```python
from build123d import *

# Parameters (mm, degrees)
SKETCH_W         = 90
SKETCH_H         = 64
PAD_DEPTH        = 2
HOLE_D           = 2.9
HOLE_DEPTH       = 25
HOLE_CSINK_D     = 6.1
HOLE_CSINK_ANGLE = 90
SKETCH002_W      = 13.6
SKETCH002_H      = 5
SKETCH002_W_2    = 5
SKETCH002_H_2    = 15
PAD001_DEPTH     = 13.6
SKETCH003_R      = 0.8
HOLE001_DEPTH    = 8
HOLE001_TIPS_R   = 0.8
SKETCH004_R      = 5
HOLE002_DEPTH    = 5
HOLE002_TIPS_R   = 5
FILLET_R         = 1


with BuildPart() as part:
    # Sketch → Pad (new body)
    with BuildSketch(Plane.XY):
        Rectangle(SKETCH_W, SKETCH_H)
    extrude(amount=PAD_DEPTH)

    # Hole
    with Locations(Plane.XY.offset(2)):
        with Locations((-40, 20), (-40, 0), (-40, -20), (40, 20), (40, 0), (40, -20)):
            CounterSinkHole(HOLE_D / 2, HOLE_CSINK_D / 2, depth=HOLE_DEPTH, counter_sink_angle=HOLE_CSINK_ANGLE)

    # Sketch002 (on Face6 of Pad) → Pad001 (join)
    with BuildSketch(Plane.XY.offset(2)):
        with Locations((-13.7, 24.6)):
            Rectangle(SKETCH002_W, SKETCH002_H)
        with Locations((-13.7, -3.4)):
            Rectangle(SKETCH002_W, SKETCH002_H)
        with Locations((32.5, 5)):
            Rectangle(SKETCH002_W_2, SKETCH002_H_2)
    extrude(amount=PAD001_DEPTH)

    # Sketch003 (on Face15 of Pad001) → Hole001 (cut)
    with BuildSketch(Plane(origin=(-20.5, 0, 0), x_dir=(0, -1, 0), z_dir=(-1, 0, 0))):
        with Locations((-24.45, 8.8)):
            Circle(SKETCH003_R)
        with Locations((3.25, 8.8)):
            Circle(SKETCH003_R)
    extrude(amount=-HOLE001_DEPTH, mode=Mode.SUBTRACT)

    # Hole001 tips → Hole001 tip 1 section 0
    with BuildSketch(Plane(origin=(-12.5, 0, 0), x_dir=(0, -1, 0), z_dir=(-1, 0, 0)), mode=Mode.PRIVATE) as hole001_tip_1_s0:
        with Locations((-24.45, 8.8)):
            Circle(HOLE001_TIPS_R)
    loft([hole001_tip_1_s0.sketch, Vertex(-12.019312, 24.45, 8.8)], mode=Mode.SUBTRACT)

    # Hole001 tips → Hole001 tip 2 section 0
    with BuildSketch(Plane(origin=(-12.5, 0, 0), x_dir=(0, -1, 0), z_dir=(-1, 0, 0)), mode=Mode.PRIVATE) as hole001_tip_2_s0:
        with Locations((3.25, 8.8)):
            Circle(HOLE001_TIPS_R)
    loft([hole001_tip_2_s0.sketch, Vertex(-12.019312, -3.25, 8.8)], mode=Mode.SUBTRACT)

    # Sketch004 (on Face28 of Hole001) → Hole002 (cut)
    with BuildSketch(Plane.YZ.offset(35)):
        with Locations((5, 8.8)):
            Circle(SKETCH004_R)
    extrude(amount=-HOLE002_DEPTH, mode=Mode.SUBTRACT)

    # Hole002 tips → Hole002 tip 1 section 0
    with BuildSketch(Plane.YZ.offset(30), mode=Mode.PRIVATE) as hole002_tip_1_s0:
        with Locations((5, 8.8)):
            Circle(HOLE002_TIPS_R)
    loft([hole002_tip_1_s0.sketch, Vertex(26.995697, 5, 8.8)], mode=Mode.SUBTRACT)

    # Fillet
    fillet_edges = [part.edges().sort_by_distance(p)[0] for p in [
        (32.5, -2.5, 15.6),
        (32.5, 12.5, 15.6),
        (-13.7, -5.9, 15.6),
        (-13.7, 27.1, 15.6),
    ]]
    fillet(fillet_edges, radius=FILLET_R)


solid = part.part
```
Input: part model. Units: mm. Frame: model coordinates. A direction names the side the tool comes from. Give positions to 0.01 mm unless a question says otherwise; leave off trailing zeros. Order: outer loops, then holes, each group sorted by start corner. A loop starts at its lowest first (then second) coordinate and runs counter-clockwise, first axis right, second up. Notation, with made-up numbers: M -1.75,-38.5 L 47.25,-38.5 A33 cw 47.25,-8.5 Z; hole C -16,20.25 d9. An arc over 180 degrees is marked long. One line per question, with ' | ' between items.
1) Section A-A on x = 40. Output: boundary loops of the cut face in (y, z).
Filled in:
outline: M -32,0 L -21.45,0 L -21.45,0.4 L -23.05,2 L -32,2 Z; M -18.55,0 L -1.45,0 L -1.45,0.4 L -3.05,2 L -16.95,2 L -18.55,0.4 Z; M 1.45,0 L 18.55,0 L 18.55,0.4 L 16.95,2 L 3.05,2 L 1.45,0.4 Z; M 21.45,0 L 32,0 L 32,2 L 23.05,2 L 21.45,0.4 Z
2) Section D-D on z = 11.5. Output: boundary loops of the cut face in (x, y).
Filled in:
outline: M -20.5,-5.9 L -6.9,-5.9 L -6.9,-0.9 L -20.5,-0.9 Z; M -20.5,22.1 L -6.9,22.1 L -6.9,27.1 L -20.5,27.1 Z; M 30,-2.5 L 35,-2.5 L 35,0.79 L 30,0.79 Z; M 30,9.21 L 35,9.21 L 35,12.5 L 30,12.5 Z
3) Contact query for flat-ended pins moving along their axis: P1, Ø2.5, axis at x = 40, y = 0, coming from the -Z side; P2, Ø2.5, axis at y = 24.45, z = 8.8, coming from the -X side; P3, Ø2.5, axis at x = 32, z = 11, coming from the -Y side; P4, Ø1.5, axis at x = 35.5, y = -21.5, coming from the +Z side. Output: stop coordinate, or through.
Filled in:
P1: passes through | P2: stops at x = -20.5 | P3: stops at y = -2.5 | P4: stops at z = 2
4) Draft query along Z for faces 5 (the face through (-14, 24, 15.6)), 6 (the face through (-1, 0, 0)), 7 (the face through (32.5, 1, 5.8)), 8 (the face through (-1, -32, 1)). Return one class per face: pulls with the +Z half, pulls with the -Z half, needs draft (parallel to the pull), parting line crosses it, or undercut.
Filled in:
face 5: pulls with the +Z half | face 6: pulls with the -Z half | face 7: undercut | face 8: needs draft
5) Section B-B on y = -20. Output: boundary loops of the cut face in (x, z).
Filled in:
outline: M -45,0 L -41.45,0 L -41.45,0.4 L -43.05,2 L -45,2 Z; M -38.55,0 L 38.55,0 L 38.55,0.4 L 36.95,2 L -36.95,2 L -38.55,0.4 Z; M 41.45,0 L 45,0 L 45,2 L 43.05,2 L 41.45,0.4 Z
6) Access query for faces 1 (the face through (-14, -5.9, 8)), 2 (the face through (30, -0.1, 10.2)), 3 (the face through (35, -0.1, 10.2)), 4 (the face through (-14, 22.1, 9)). Directions: +Z, -Z, +X, -X, +Y, -Y. A direction counts if a zero-diameter tool reaches every point of the face in a straight line with its end or side. Return the directions, or none.
Filled in:
face 1: +Z, +X, -X, -Y | face 2: +Z, +Y, -Y | face 3: +Z, +X, +Y, -Y | face 4: +Z, +X, -X
7) Ray query, L1, parallel to Y at x = 40, z = 0.2; L2, parallel to X at y = 20, z = 0.25; L3, parallel to Z at x = -18, y = -3.25. Return the intervals inside material, ascending.
Filled in:
L1: y = -32 to -21.45, -18.55 to -1.45, 1.45 to 18.55, 21.45 to 32 | L2: x = -45 to -41.45, -38.55 to 38.55, 41.45 to 45 | L3: z = 0 to 8, 9.6 to 15.6
8) Section C-C on y = 4. Output: boundary loops of the cut face in (x, z), and give its area (3 significant figures).
Filled in:
outline: M -45,0 L 45,0 L 45,2 L 35,2 L 35,3.9 L 30,3.9 L 30,2 L -45,2 Z; M 30,13.7 L 35,13.7 L 35,15.6 L 30,15.6 Z | area: 199 mm2
